Answer from the drawing. Dimensions are ordinates in mm from the lowest x, y and z of the part. Give positions to 0.01 mm unless a question says otherwise; leave off trailing zeros. Order: outer loops, then holes, each group sorted by start corner. A loop starts at its lowest first (then second) coordinate and runs counter-clockwise, first axis right, second up. Notation, with made-up numbers: (-4, -24) - (53, -24) arc R22 cw to (53, -10) - close; hole circle Ø9 at (-28.75, -5). An arc over 180 degrees is marked (long way). Answer in a Markdown table with one row per item.
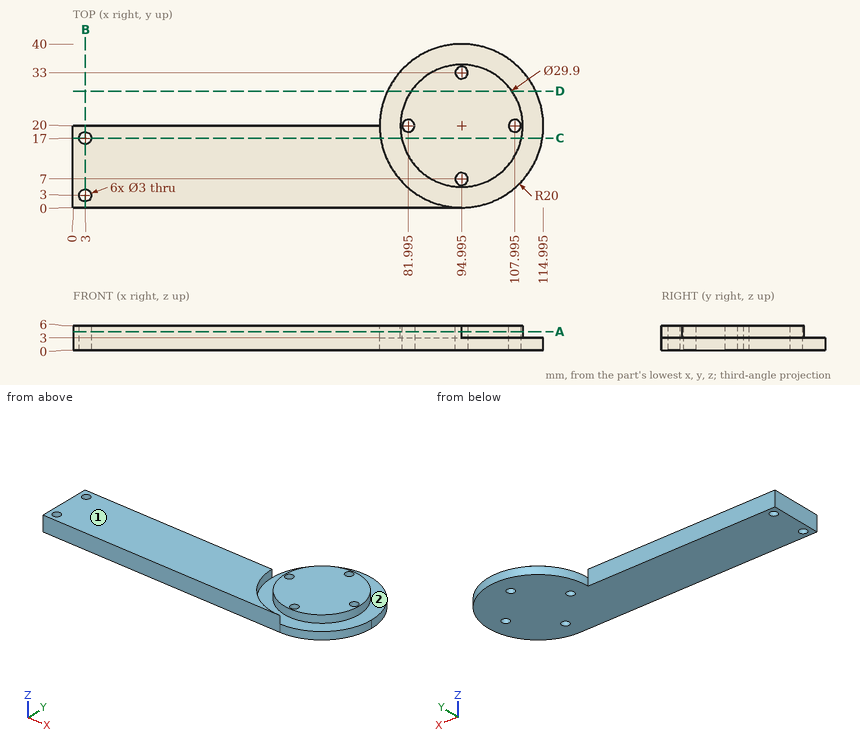
Item 1: Find section B-B on x = 3. Write down the section's boundary in (y, z).
Answer block:
| item | result |
|---|---|
| outline | (0, 0) - (1.5, 0) - (1.5, 6) - (0, 6) - close; (4.5, 0) - (15.5, 0) - (15.5, 6) - (4.5, 6) - close; (18.5, 0) - (20, 0) - (20, 6) - (18.5, 6) - close |
Item 2: Determine the mould class of the marked faces 1 and 2 for opening direction Y: pulls with the +Y half, pulls with the -Y half, needs draft (parallel to the pull), parting line crosses it, or undercut.
Answer block:
| item | result |
|---|---|
| face 1 | needs draft |
| face 2 | undercut |
Item 3: Consider line 1 (Y direction, x = 3, z = 1.35); line 2 (Y direction, x = 63.5, z = 2.4); line 3 (Z direction, x = 105.5, y = 32). Determine where each line is inside the solid, lowest interval first.
Answer block:
| item | result |
|---|---|
| line 1 | 0 to 1.5, 4.5 to 15.5, 18.5 to 20 |
| line 2 | 0 to 20 |
| line 3 | 0 to 3 |
Item 4: Each of these flat-tipped pins is pushed along its axis until it touches: P1, Ø3, axis at x = 29.5, z = 4, coming from the +Y side; P2, Ø1.5, axis at y = 33.5, z = 5.5, coming from the +X side. Where does it stop, or does it pass through?
Answer block:
| item | result |
|---|---|
| P1 | y = 20 |
| P2 | x = 102.8 |
Item 5: Find section A-A on z = 4.5. Write down the section's boundary in (x, y) (3 decimals), then the cut area to 3 significant figures.
Answer block:
| item | result |
|---|---|
| outline | (0, 0) - (94.995, 0) arc R20 cw to (74.995, 20) - (0, 20) - close; circle Ø29.9 at (94.995, 20); hole circle Ø3 at (3, 3); hole circle Ø3 at (3, 17); hole circle Ø3 at (81.995, 20); hole circle Ø3 at (94.995, 7); hole circle Ø3 at (94.995, 33); hole circle Ø3 at (107.995, 20) |
| area | 2,250 mm² |
Item 6: Find section C-C on y = 17. Write down the section's boundary in (x, z), then the cut area to 3 significant figures.
Answer block:
| item | result |
|---|---|
| outline | (0, 0) - (1.5, 0) - (1.5, 6) - (0, 6) - close; (4.5, 0) - (114.77, 0) - (114.77, 3) - (109.64, 3) - (109.64, 6) - (80.35, 6) - (80.35, 3) - (75.22, 3) - (75.22, 6) - (4.5, 6) - close |
| area | 640 mm² |
Item 7: Find section D-D on y = 28.5. Write down the section's boundary in (x, z).
Answer block:
| item | result |
|---|---|
| outline | (76.89, 0) - (113.1, 0) - (113.1, 3) - (107.29, 3) - (107.29, 6) - (82.7, 6) - (82.7, 3) - (76.89, 3) - close |
